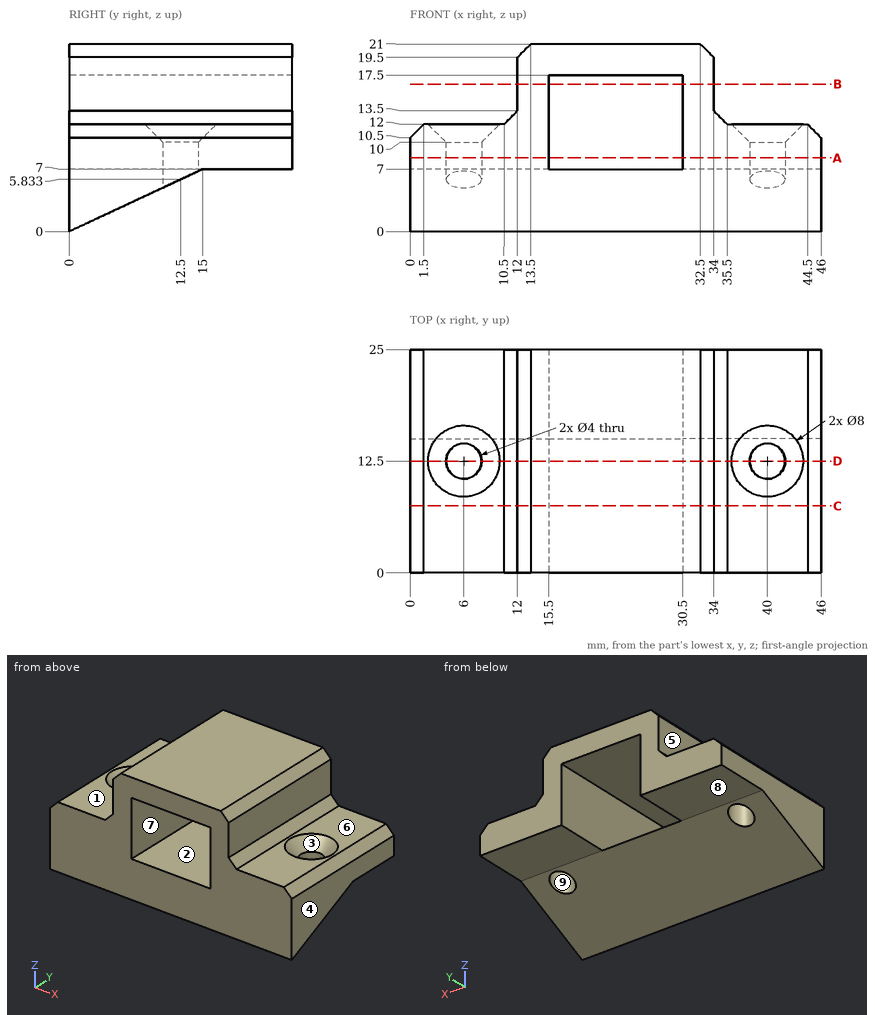
Study the drawing (mm; zero at the part's minimum x, y, z) and answer. A direction names the side the tool comes from. Give positions to 0.01 mm unless a question says otherwise; leave off trailing zeros. Order: outer loops, then holes, each group sorted by start corner. A loop starts at its lowest first (then second) coordinate and runs counter-clockwise, first axis right, second up. Notation, with made-up numbers: (-37, 44) -> (3, 44) arc R23 ccw to (3, 75) -> close; hole circle Ø10 at (-20.5, 66). An arc over 180 degrees is marked (long way). Write item = value, one per line.
1. A cutting plane is placed at D-D, the plane y = 12.5. Count the separate pieces of the cut face and the enclosed holes in it.
Numbers:
separate_pieces = 3
enclosed_holes = 1
2. A cutting plane is placed at B-B, the plane z = 16.5. Write down the section's boundary in (x, y).
Numbers:
outline = (12, 0) -> (15.5, 0) -> (15.5, 25) -> (12, 25) -> close; (30.5, 0) -> (34, 0) -> (34, 25) -> (30.5, 25) -> close
3. A cutting plane is placed at C-C, the plane y = 7.5. Write down the section's boundary in (x, z).
Numbers:
outline = (0, 3.5) -> (46, 3.5) -> (46, 10.5) -> (44.5, 12) -> (35.5, 12) -> (34, 13.5) -> (34, 19.5) -> (32.5, 21) -> (13.5, 21) -> (12, 19.5) -> (12, 13.5) -> (10.5, 12) -> (1.5, 12) -> (0, 10.5) -> close; hole (15.5, 7) -> (30.5, 7) -> (30.5, 17.5) -> (15.5, 17.5) -> close
4. Straight lines are drawn through the part: line 1 along Y through (x, z) = (40, 8.2); line 2 along X through (y, z) = (19.75, 9); line 3 along Z through (x, y) = (36, 20.5). For each, find the intervals that lie inside material, in ascending order.
Numbers:
line_1 = 0 to 10.5, 14.5 to 25
line_2 = 0 to 15.5, 30.5 to 46
line_3 = 7 to 12
5. For the marked faces 5, 6, 7, 8 and 9, determine the directions among +Z, -Z, +X, -X, +Y, -Y from which every point of the face is accessible in a straight line to the end or side of a thin tool.
Numbers:
face_5 = +Z, -X, +Y, -Y
face_6 = +Z, +X, +Y, -Y
face_7 = +Y, -Y
face_8 = -Z, +X, -X, +Y
face_9 = +Z, -Z
6. The mould has two halves that part along X. Classify the marked faces 1, 2, 3 and 4: +X half, -X half, draft (parallel to the pull), parting line (faces both ways), or undercut.
Numbers:
face_1 = draft
face_2 = undercut
face_3 = undercut
face_4 = +X half
7. A cutting plane is placed at A-A, the plane z = 8.25. Write down the section's boundary in (x, y), and give its area (3 significant figures).
Numbers:
outline = (0, 0) -> (15.5, 0) -> (15.5, 25) -> (0, 25) -> close; (30.5, 0) -> (46, 0) -> (46, 25) -> (30.5, 25) -> close; hole circle Ø4 at (6, 12.5); hole circle Ø4 at (40, 12.5)
area = 750 mm²
8. Given pin 1 (3 mm diameter, centred on x = 39.5, y = 21.5, fed in from -Z); pin 2 (12 mm diameter, centred on x = 25.5, y = 12.5, fed in from -Z); pin 3 (7 mm diameter, centred on x = 7.5, y = 16.5, fed in from +Z); pin 4 (2.5 mm diameter, centred on x = 6, y = 12.5, fed in from +Z), each flat-ended and moving along its own axis, determine where each tip first touches the part or whether it passes through.
Numbers:
pin_1 = 7
pin_2 = 3.03
pin_3 = 12.5
pin_4 = through
